For this review, take the finished solid that the model builds, in its own axes (mm). A direction names the side the tool comes from. Give positions to 0.01 mm unless a question says otherwise; leave off trailing zeros. Write each loop counter-clockwise with the first axis right and the second up, starting at its lowest first coordinate (ties: lowest second). Pieces come first, ordered by that corner, then holes.
1) We need section D-D on z = -4.75. Give the boundary of the cut face in (x, y), and give its area (3 significant figures).
2) We need section A-A on z = -13. Give the boundary of the cut face in (x, y).
3) Wall thickness on line 1 along Y through (x, z) = (13.2, -1.55); line 2 along Y through (x, z) = (0.55, -5); line 3 along Y through (x, z) = (1.15, -13): over which ranges is each line inside the solid? List them lowest first.
4) Machinability: for faces 5 (the face through (1.01, 10.74, -12.84)), 6 (the face through (2, 22, -9)), which of the approach directions +Z, -Z, +X, -X, +Y, -Y give a long, thin tool a straight path to every point of the face, cutting with its end or side? Answer none if there is none.
5) Draft analysis for pull direction Y (two halves, no side actions). For faces 1 (the face through (4.4, 0, -1.5)), 2 (the face through (12.623, 4.891, -1.014)), 3 (the face through (1.01, 14.74, -4.84)), 4 (the face through (0, 22, -8)), state which applies: pulls with the +Y half, pulls with the -Y half, needs draft (parallel to the pull), parting line crosses it, or undercut.
6) For P1, Ø4, axis at x = 6.5, z = -5.5, coming from the +Y side; P2, Ø4, axis at y = 33.5, z = -9.5, coming from the +X side; P3, Ø1, axis at x = 4.5, y = 9.5, coming from the -Z side, all flat-tipped, find the tip position at first contact; note any pin that passes through.
7) We need section B-B on x = 13.2. Give the boundary of the cut face in (y, z), and give its area (3 significant figures).
8) We need section C-C on y = 37. Give the boundary of the cut face in (x, z), and give its area (3 significant figures).
from build123d import *

# Parameters (mm, degrees)
BOSS_EXTRUDE1_DEPTH = 45
SKETCH2_R           = 1.25
CUT_EXTRUDE1_DEPTH  = 50.769468553
SKETCH3_R           = 1.25
CUT_EXTRUDE2_DEPTH  = 50.769468553


with BuildPart() as part:
    # Sketch1 → Boss-Extrude1 (new body)
    with BuildSketch(Plane(origin=(0, 0, 0), x_dir=(1, 0, 0), z_dir=(0, 1, 0))):
        Polygon((0, 0), (16, 0), (16, 2), (2, 2), (2, 16), (0, 16), align=None)
    extrude(amount=BOSS_EXTRUDE1_DEPTH)

    # Sketch2 → Cut-Extrude1 (cut, through all)
    with BuildSketch(Plane(origin=(0, 0, -2), x_dir=(-1, 0, 0), z_dir=(0, 0, -1))):
        with Locations((-13.2, 37)):
            Circle(SKETCH2_R)
        with Locations((-13.2, 6)):
            Circle(SKETCH2_R)
    extrude(amount=-CUT_EXTRUDE1_DEPTH, mode=Mode.SUBTRACT)

    # Sketch3 → Cut-Extrude2 (cut, through all)
    with BuildSketch(Plane(origin=(2, 0, 0), x_dir=(0, 0, -1), z_dir=(1, 0, 0))):
        with Locations((13, 9.5)):
            Circle(SKETCH3_R)
        with Locations((5, 13.5)):
            Circle(SKETCH3_R)
    extrude(amount=-CUT_EXTRUDE2_DEPTH, mode=Mode.SUBTRACT)


solid = part.part
Results list:
1. outline: (0, 0) - (2, 0) - (2, 12.28) - (0, 12.28) - close; (0, 14.72) - (2, 14.72) - (2, 45) - (0, 45) - close
1. area: 85.1 mm2
2. outline: (0, 0) - (2, 0) - (2, 8.25) - (0, 8.25) - close; (0, 10.75) - (2, 10.75) - (2, 45) - (0, 45) - close
3. line 1: y = 0 to 4.75, 7.25 to 35.75, 38.25 to 45
3. line 2: y = 0 to 12.25, 14.75 to 45
3. line 3: y = 0 to 8.25, 10.75 to 45
4. face 5: +X, -X
4. face 6: -Z, +X, +Y, -Y
5. face 1: pulls with the -Y half
5. face 2: undercut
5. face 3: undercut
5. face 4: needs draft
6. P1: passes through
6. P2: stops at x = 2
6. P3: stops at z = -2
7. outline: (0, -2) - (4.75, -2) - (4.75, 0) - (0, 0) - close; (7.25, -2) - (35.75, -2) - (35.75, 0) - (7.25, 0) - close; (38.25, -2) - (45, -2) - (45, 0) - (38.25, 0) - close
7. area: 80.0 mm2
8. outline: (0, -16) - (2, -16) - (2, -2) - (11.95, -2) - (11.95, 0) - (0, 0) - close; (14.45, -2) - (16, -2) - (16, 0) - (14.45, 0) - close
8. area: 55.0 mm2
